Read the model definition and answer for the solid it produces. Units are mm, in the model's axes. Coordinates: 2 decimals unless noted, no trailing zeros. Write each loop counter-clockwise with the first axis right and the second up, starting at its lowest first coordinate (ties: lowest second). Pieces come first, ordered by that corner, then holes. Notation, with made-up numbers: (38, -1.75) -> (73, -1.75) arc R22 ccw to (73, 16.25) -> close; hole circle Ø1 at (61, 65). An arc over 180 degrees is marked (long way). Use CSV: the item, a comma, the result in double quotes.
from build123d import *

# Parameters (mm, degrees)
SKETCH1_R           = 2.5
BOSS_EXTRUDE1_DEPTH = 1


with BuildPart() as part:
    # Sketch1 → Boss-Extrude1 (new body)
    with BuildSketch(Plane(origin=(0, 0, 0), x_dir=(1, 0, 0), z_dir=(0, 1, 0))):
        Polygon((20.6, 50), (40.6, 50), (40.6, -50), (20.6, -50), (-0.238673257, -27.92), (-18, -27.92), (-40.6, -3.973753814), (-40.6, 3.973753814), (-18, 27.92), (-0.238673257, 27.92), align=None)
        with Locations((-30.6, 0)):
            Circle(SKETCH1_R, mode=Mode.SUBTRACT)
        with Locations((30.6, 40)):
            Circle(SKETCH1_R, mode=Mode.SUBTRACT)
        with Locations((30.6, -40)):
            Circle(SKETCH1_R, mode=Mode.SUBTRACT)
        with Locations((9.42, 0)):
            Circle(SKETCH1_R, mode=Mode.SUBTRACT)
        with Locations((-11, 0)):
            Circle(SKETCH1_R, mode=Mode.SUBTRACT)
    extrude(amount=BOSS_EXTRUDE1_DEPTH)


solid = part.part
1. Find the intervals of material crossed by line 1 along Z through (x, y) = (30.6, 0.5); line 2 along X through (y, z) = (0.55, 0); line 3 along X through (y, z) = (0.9, -0.5), in increasing order.
Solutions:
line 1,"z = -50 to -42.5, -37.5 to 37.5, 42.5 to 50"
line 2,"x = -40.6 to -33.1, -28.1 to -13.5, -8.5 to 6.92, 11.92 to 40.6"
line 3,"x = -40.6 to -33.05, -28.15 to -13.45, -8.55 to 6.97, 11.87 to 40.6"
2. A cutting plane is placed at C-C (y = 0.8). Give the vertices of the cut face in (x, z).
Solutions:
outline,"(-40.6, -3.97) -> (-18, -27.92) -> (-0.24, -27.92) -> (20.6, -50) -> (40.6, -50) -> (40.6, 50) -> (20.6, 50) -> (-0.24, 27.92) -> (-18, 27.92) -> (-40.6, 3.97) -> close; hole circle Ø5 at (-30.6, 0); hole circle Ø5 at (-11, 0); hole circle Ø5 at (9.42, 0); hole circle Ø5 at (30.6, -40); hole circle Ø5 at (30.6, 40)"
3. A cutting plane is placed at D-D (x = 30.6). Give the vertices of the cut face in (y, z).
Solutions:
outline,"(0, -50) -> (1, -50) -> (1, -42.5) -> (0, -42.5) -> close; (0, -37.5) -> (1, -37.5) -> (1, 37.5) -> (0, 37.5) -> close; (0, 42.5) -> (1, 42.5) -> (1, 50) -> (0, 50) -> close"
4. A cutting plane is placed at A-A (x = -11). Give the vertices of the cut face in (y, z), and give its area (3 significant figures).
Solutions:
outline,"(0, -27.92) -> (1, -27.92) -> (1, -2.5) -> (0, -2.5) -> close; (0, 2.5) -> (1, 2.5) -> (1, 27.92) -> (0, 27.92) -> close"
area,"50.8 mm^2"
5. A cutting plane is placed at B-B (z = 0). Give the vertices of the cut face in (x, y).
Solutions:
outline,"(-40.6, 0) -> (-33.1, 0) -> (-33.1, 1) -> (-40.6, 1) -> close; (-28.1, 0) -> (-13.5, 0) -> (-13.5, 1) -> (-28.1, 1) -> close; (-8.5, 0) -> (6.92, 0) -> (6.92, 1) -> (-8.5, 1) -> close; (11.92, 0) -> (40.6, 0) -> (40.6, 1) -> (11.92, 1) -> close"
6. For a pull along Z with two mould halves and no side action, classify faces 1 (the cylindrical face through (6.922, 0.493, -0.11)), 2 (the flat face through (-29.46, 0.49, -15.78)), 3 (the flat face through (10.327, 0.493, 39.115)) as pulls with the +Z half, pulls with the -Z half, needs draft (parallel to the pull), parting line crosses it, or undercut.
Solutions:
face 1,"undercut"
face 2,"pulls with the -Z half"
face 3,"pulls with the +Z half"
7. This flat-tipped pin is pushed along its axis until it touches: pin 1 Ø4 at (x, z) = (-30.6, 0) entering from +Y. Where does it stop, or does it pass through?
Solutions:
pin 1,"passes through"
